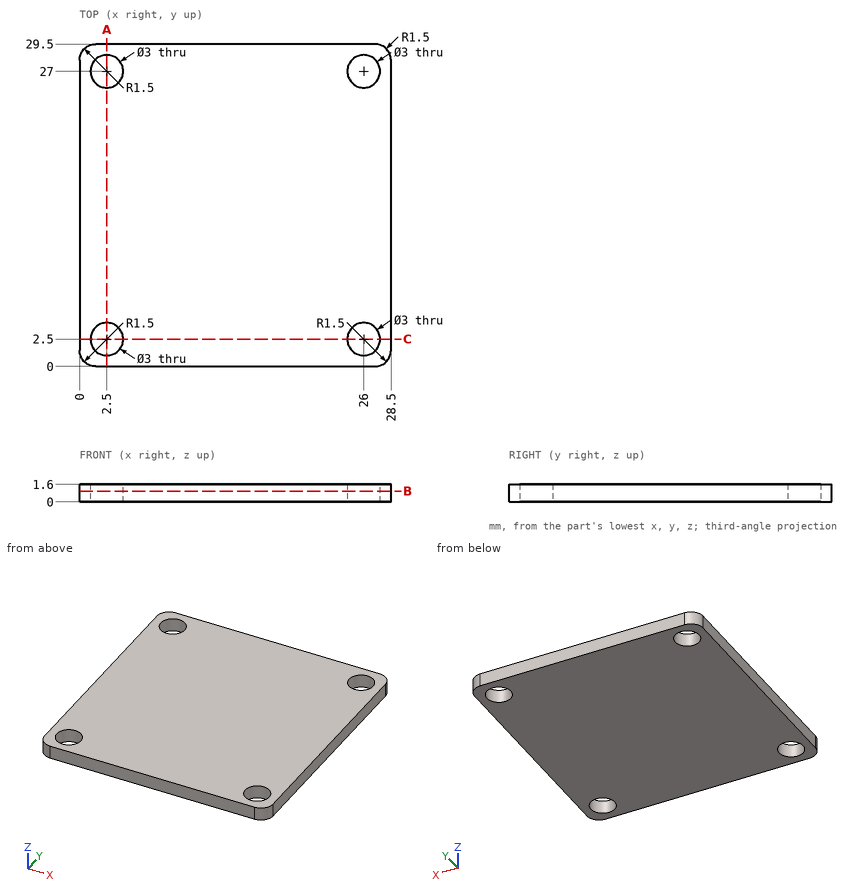
Study the drawing (mm; zero at the part's minimum x, y, z) and answer. Coordinates: 2 decimals unless noted, no trailing zeros. Order: outer loops, then holes, each group sorted by start corner. A loop starts at its lowest first (then second) coordinate and runs counter-clockwise, first axis right, second up. Notation, with made-up numbers: M -39.5,-40 L 13.5,-40 A26 ccw 13.5,-22 Z; hole C 9.25,55.25 d11. An arc over 180 degrees is marked long. Answer as a JSON object with one key per item and string values. Group by question number.
1. A flat-ended cylindrical pin translates along its axis: P1, Ø1.8, axis at x = 2.5, y = 27, coming from the +Z side. Find the tip coordinate at first contact, or state that the pin passes through.
2. Section C-C on y = 2.5 is taken. Write down the section's boundary in (x, z), then the cut area to 3 significant figures.
3. Section A-A on x = 2.5 is taken. Write down the section's boundary in (y, z).
4. Section B-B on z = 1 is taken. Write down the section's boundary in (x, y), then the cut area to 3 significant figures.
5. Straight lines are drawn through the part: line 1 (Y direction, x = 2.5, z = 0.85); line 2 (X direction, y = 2.25, z = 1.3); line 3 (Y direction, x = 1.75, z = 0.2). For each, find the intervals that lie inside material, in ascending order.
Values follow:
{
 "1": {"P1": "through"},
 "2": {"outline": "M 0,0 L 1,0 L 1,1.6 L 0,1.6 Z; M 4,0 L 24.5,0 L 24.5,1.6 L 4,1.6 Z; M 27.5,0 L 28.5,0 L 28.5,1.6 L 27.5,1.6 Z", "area": "36.0 mm2"},
 "3": {"outline": "M 0,0 L 1,0 L 1,1.6 L 0,1.6 Z; M 4,0 L 25.5,0 L 25.5,1.6 L 4,1.6 Z; M 28.5,0 L 29.5,0 L 29.5,1.6 L 28.5,1.6 Z"},
 "4": {"outline": "M 0,1.5 A1.5 ccw 1.5,0 L 27,0 A1.5 ccw 28.5,1.5 L 28.5,28 A1.5 ccw 27,29.5 L 1.5,29.5 A1.5 ccw 0,28 Z; hole C 2.5,2.5 d3; hole C 2.5,27 d3; hole C 26,2.5 d3; hole C 26,27 d3", "area": "811 mm2"},
 "5": {"line 1": "0 to 1, 4 to 25.5, 28.5 to 29.5", "line 2": "0 to 1.02, 3.98 to 24.52, 27.48 to 28.5", "line 3": "0 to 1.2, 3.8 to 25.7, 28.3 to 29.5"}
}
